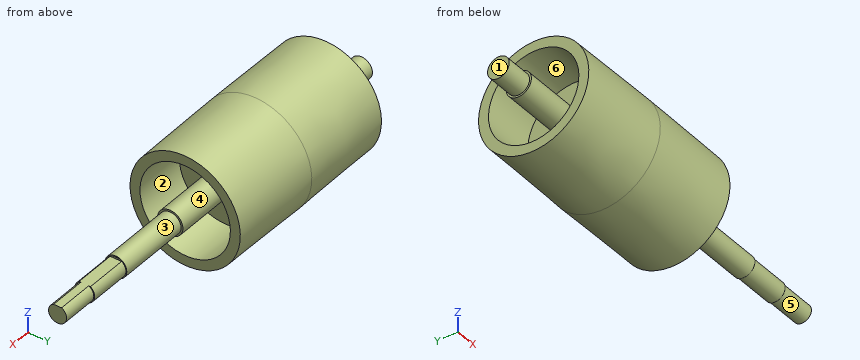
```python
from build123d import *

# Parameters (mm, degrees)
F4_W     = 43.39286
F4_H     = 11.136995
F5_DEPTH = 1


with BuildPart() as f1:
    # F0 (on Front) → F1 (revolve)
    with BuildSketch(Plane.XZ):
        Polygon((-52.789021, 6), (-52.789021, 0), (171.210979, 0), (171.210979, 5), (151.210979, 5), (151.210979, 5.5), (128.210979, 5.5), (128.210979, 6), (88.210979, 6), (88.210979, 7), (48.210979, 7), (48.210979, 25), (77.210979, 25), (77.210979, 30.5), (25.210979, 31), (-26.789021, 30.5), (-26.789021, 25), (2.210979, 25), (2.210979, 7), (-37.789021, 7), (-37.789021, 6), align=None)
    revolve(axis=Axis((59.210979, 0, 0), (-1, 0, 0)))


with BuildPart() as f1_1:
    # F3: moved
    add(f1.part.moved(Location((-70, 0, 0))))

    # F4 (on offset) → F5 (cut)
    with BuildSketch(Plane.XY.offset(5.5)):
        with Locations((80.00974, 0.016809)):
            Rectangle(F4_W, F4_H)
    extrude(amount=-F5_DEPTH, mode=Mode.SUBTRACT)


solid = f1_1.part
```
Can you work these out from the model? Positions are in its coordinate system, mm. Face numbers are marked on the shaded views. A direction names the side the tool comes from. Coordinates: 2 decimals unless noted, no trailing zeros. Loops run counter-clockwise (first coordinate to the right, second up) from the corner with the lowest first, then second, coordinate; pieces in that order, holes last.
Item 1: Suppose I cut it at A-A (x = -77). Please give me the cut outline in (y, z).
Answers below:
outline: circle Ø61.38 at (0, 0); circle Ø14 at (0, 0); hole circle Ø50 at (0, 0)
Item 2: If we mould it in two halves opening along Z, with no side actions, what happens to the marked faces 1, 2, 3 and 4? For each: released by +Z, released by -Z, zero draft, split by the parting line, or undercut.
Answers below:
face 1: zero draft
face 2: undercut
face 3: split by the parting line
face 4: undercut
Item 3: I'm going to push flat-ended pins straight in: pin 1 (3 mm diameter, centred on y = -1, z = -19.5, fed in from -X); pin 2 (2 mm diameter, centred on y = 6.5, z = 6.5, fed in from +X); pin 3 (10 mm diameter, centred on x = -61, z = -20.5, fed in from -Y). Where does each tip first touch, or does it pass through?
Answers below:
pin 1: stops at x = -67.79
pin 2: stops at x = -21.79
pin 3: stops at y = -26.67
Item 4: Suppose I cut it at C-C (x = -34.5). Please give me the cut outline in (y, z).
Answers below:
outline: circle Ø61.8 at (0, 0)
Item 5: Suppose I cut it at B-B (x = 84.5). Please give me the cut outline in (y, z), then the cut area to 3 significant figures.
Answers below:
outline: (-2.18, 4.5) arc R5 ccw (long way) to (2.18, 4.5) - close
area: 77.1 mm2
Item 6: Please list where these lines run through material, in increasing order: L1, parallel to Y at x = -13.5, z = 0; L2, parallel to X at y = 12, z = -27; L3, parallel to Z at x = 71, y = 0.
Answers below:
L1: y = -30.7 to -25, -7 to 7, 25 to 30.7
L2: x = -96.79 to 7.21
L3: z = -5.5 to 4.5
Item 7: Which directions (+Z, -Z, +X, -X, +Y, -Y) give clear straight access to the entire face, cutting with the end or side of a thin tool? Please do the marked faces 5 and 6.
Answers below:
face 5: +X
face 6: -X
